```python
from build123d import *

# Parameters (mm, degrees)
PRISM003_DEPTH         = 6
PRISM002_DEPTH         = 6
BOX004_W               = 10
BOX004_H               = 12
BOX004_DEPTH           = 4
BOX003_W               = 35
BOX003_H               = 26.5
BOX003_DEPTH           = 10
BOX002_W               = 70
BOX002_H               = 19
BOX002_DEPTH           = 19
BOX002_PLACEMENT_ANGLE = 30
BOX001_W               = 70
BOX001_H               = 19
BOX001_DEPTH           = 19
BOX001_PLACEMENT_ANGLE = 90.0000000001
BOX_W                  = 70
BOX_H                  = 19
BOX_DEPTH              = 19
BOX_PLACEMENT_ANGLE    = 30
PRISM001_DEPTH         = 25
PRISM_DEPTH            = 25
FILLET_R               = 15
SKETCH001_R            = 2
POCKET_DEPTH           = 782.7773522307
POLARPATTERN_COUNT     = 3
POCKET001_DEPTH        = 3
SKETCH002_R            = 1
POCKET002_DEPTH        = 782.7773522307
POLARPATTERN001_COUNT  = 3
SKETCH004_R            = 1
POCKET003_DEPTH        = 782.7773522307
POLARPATTERN002_COUNT  = 3
POLARPATTERN003_COUNT  = 3
SKETCH005_R            = 1
POCKET004_DEPTH        = 782.7773522307
POLARPATTERN004_COUNT  = 3
POCKET005_DEPTH        = 22.001
SKETCH007_W            = 14
SKETCH007_H            = 9
POCKET006_DEPTH        = 20


with BuildPart() as prism003:
    # Prism003 → Prism003 (new body)
    with BuildSketch(Plane.XY.offset(13)):
        Polygon((106, 0), (-53, 91.7986928012), (-53, -91.7986928012), align=None)
    extrude(amount=PRISM003_DEPTH)


with BuildPart() as cut006:
    # Prism002 → Prism002 (new body)
    with BuildSketch(Plane.XY.offset(13)):
        Polygon((152, 0), (-76, 131.6358613752), (-76, -131.6358613752), align=None)
    extrude(amount=PRISM002_DEPTH)

    # Cut006: cut Prism003
    add(prism003.part, mode=Mode.SUBTRACT)


with BuildPart() as box004:
    # Box004 → Box004 (new body)
    with BuildSketch(Plane(origin=(84, -6, 15), x_dir=(1, 0, 0), z_dir=(0, 0, 1))):
        with Locations((5, 6)):
            Rectangle(BOX004_W, BOX004_H)
    extrude(amount=BOX004_DEPTH)


with BuildPart() as box003:
    # Box003 → Box003 (new body)
    with BuildSketch(Plane(origin=(93, -13.3, 9), x_dir=(1, 0, 0), z_dir=(0, 0, 1))):
        with Locations((17.5, 13.25)):
            Rectangle(BOX003_W, BOX003_H)
    extrude(amount=BOX003_DEPTH)


with BuildPart() as box002:
    # Box002 → Box002 (new body)
    with BuildSketch(Plane.XY):
        with Locations((35, 9.5)):
            Rectangle(BOX002_W, BOX002_H)
    extrude(amount=BOX002_DEPTH)


with BuildPart() as box002_1:
    # Box002 placement: moved
    add(box002.part.moved(Location((7, -82, 0))).rotate(Axis((7, -82, 0), (0, 0, 1)), BOX002_PLACEMENT_ANGLE))


with BuildPart() as box001:
    # Box001 → Box001 (new body)
    with BuildSketch(Plane.XY):
        with Locations((35, 9.5)):
            Rectangle(BOX001_W, BOX001_H)
    extrude(amount=BOX001_DEPTH)


with BuildPart() as box001_1:
    # Box001 placement: moved
    add(box001.part.moved(Location((-55, -35, 0))).rotate(Axis((-55, -35, 0), (0, 0, 1)), BOX001_PLACEMENT_ANGLE))


with BuildPart() as box:
    # Box → Box (new body)
    with BuildSketch(Plane.XY):
        with Locations((35, 9.5)):
            Rectangle(BOX_W, BOX_H)
    extrude(amount=BOX_DEPTH)


with BuildPart() as box_1:
    # Box placement: moved
    add(box.part.moved(Location((-2, 65, 0))).rotate(Axis((-2, 65, 0), (0, 0, -1)), BOX_PLACEMENT_ANGLE))


with BuildPart() as prism001:
    # Prism001 → Prism001 (new body)
    with BuildSketch(Plane.XY.offset(-6)):
        Polygon((95, 0), (-47.5, 82.2724133595), (-47.5, -82.2724133595), align=None)
    extrude(amount=PRISM001_DEPTH)


with BuildPart() as body:
    # Prism → Prism (new body)
    with BuildSketch(Plane.XY.offset(-6)):
        Polygon((165, 0), (-82.5, 142.8941916244), (-82.5, -142.8941916244), align=None)
    extrude(amount=PRISM_DEPTH)

    # Cut: cut Prism001
    add(prism001.part, mode=Mode.SUBTRACT)

    # Cut001: cut Box
    add(box_1.part, mode=Mode.SUBTRACT)

    # Cut002: cut Box001
    add(box001_1.part, mode=Mode.SUBTRACT)

    # Cut003: cut Box002
    add(box002_1.part, mode=Mode.SUBTRACT)

    # Cut004: cut Box003
    add(box003.part, mode=Mode.SUBTRACT)

    # Cut005: cut Box004
    add(box004.part, mode=Mode.SUBTRACT)

    # Cut007: cut Cut006
    add(cut006.part, mode=Mode.SUBTRACT)

    # Fillet
    fillet_edges = [body.edges().sort_by_distance(p)[0] for p in [
        (152, 0, 16),
        (-76, 131.635861, 16),
        (-76, -131.635861, 16),
    ]]
    fillet(fillet_edges, radius=FILLET_R)

    # Sketch001 (on Face1 of BaseFeature) → Pocket (cut, through all)
    with BuildSketch(Plane.XY.offset(19)):
        with Locations((148.549835, 0)):
            Circle(SKETCH001_R)
    pocket = extrude(amount=-POCKET_DEPTH, mode=Mode.SUBTRACT)

    # PolarPattern: Pocket ×3 about axis
    polarpattern_axis = Axis((0, 0, 19), (0, 0, 1))
    for i in range(1, POLARPATTERN_COUNT):
        add(pocket.rotate(polarpattern_axis, i * 360 / POLARPATTERN_COUNT), mode=Mode.SUBTRACT)

    # Sketch003 (on Face14 of PolarPattern) → Pocket001 (cut)
    with BuildSketch(Plane(origin=(0, 0, -6), x_dir=(1, 0, 0), z_dir=(0, 0, -1))):
        Polygon((-70.5, 122.1095819336), (141, 0), (-70.5, -122.1095819336), align=None)
        Polygon((-59.5, -103.0570230503), (-59.5, 103.0570230503), (119, 0), align=None, mode=Mode.SUBTRACT)
    extrude(amount=-POCKET001_DEPTH, mode=Mode.SUBTRACT)

    # Sketch002 (on Face39 of PolarPattern) → Pocket002 (cut, through all)
    with BuildSketch(Plane.XY.offset(19)):
        with Locations((-50.25, 0)):
            Circle(SKETCH002_R)
        with Locations((-50.25, 87.0355530803)):
            Circle(SKETCH002_R)
    pocket002 = extrude(amount=-POCKET002_DEPTH, mode=Mode.SUBTRACT)

    # PolarPattern001: Pocket002 ×3 about axis
    polarpattern001_axis = Axis((0, 0, 19), (0, 0, 1))
    for i in range(1, POLARPATTERN001_COUNT):
        add(pocket002.rotate(polarpattern001_axis, i * 360 / POLARPATTERN001_COUNT), mode=Mode.SUBTRACT)

    # Sketch004 (on Face40 of PolarPattern001) → Pocket003 (cut, through all)
    with BuildSketch(Plane.XY.offset(19)):
        with Locations((84.4115427319, 9)):
            Circle(SKETCH004_R)
        with Locations((84.4115427319, -9)):
            Circle(SKETCH004_R)
    pocket003 = extrude(amount=-POCKET003_DEPTH, mode=Mode.SUBTRACT)

    # PolarPattern002: Pocket003 ×3 about axis
    polarpattern002_axis = Axis((0, 0, 19), (0, 0, 1))
    for i in range(1, POLARPATTERN002_COUNT):
        add(pocket003.rotate(polarpattern002_axis, i * 360 / POLARPATTERN002_COUNT), mode=Mode.SUBTRACT)

    # PolarPattern003: Pocket002 ×3 about axis
    polarpattern003_axis = Axis((0, 0, 19), (0, 0, 1))
    for i in range(1, POLARPATTERN003_COUNT):
        add(pocket002.rotate(polarpattern003_axis, i * 360 / POLARPATTERN003_COUNT), mode=Mode.SUBTRACT)

    # Sketch005 (on Face1 of PolarPattern003) → Pocket004 (cut, through all)
    with BuildSketch(Plane.XY.offset(19)):
        with Locations((-79.25, 0)):
            Circle(SKETCH005_R)
    pocket004 = extrude(amount=-POCKET004_DEPTH, mode=Mode.SUBTRACT)

    # PolarPattern004: Pocket004 ×3 about axis
    polarpattern004_axis = Axis((0, 0, 19), (0, 0, 1))
    for i in range(1, POLARPATTERN004_COUNT):
        add(pocket004.rotate(polarpattern004_axis, i * 360 / POLARPATTERN004_COUNT), mode=Mode.SUBTRACT)

    # Sketch006 (on Face42 of PolarPattern004) → Pocket005 (cut, through all)
    with BuildSketch(Plane(origin=(0, 0, -3), x_dir=(1, 0, 0), z_dir=(0, 0, -1))):
        with BuildLine():
            ThreePointArc((123, 1.5), (121.5, 0), (123, -1.5))
            Line((123, -1.5), (135, -1.5))
            ThreePointArc((135, -1.5), (136.5, 0), (135, 1.5))
            Line((123, 1.5), (135, 1.5))
        make_face()
    extrude(amount=-POCKET005_DEPTH, mode=Mode.SUBTRACT)

    # Sketch007 (on Face3 of Pocket005) → Pocket006 (cut)
    with BuildSketch(Plane(origin=(41.25, -71.4470958122, 0), x_dir=(0.8660254038, 0.5, 0), z_dir=(0.5, -0.8660254038, 0))):
        with Locations((57.9152, 9.460156)):
            Rectangle(SKETCH007_W, SKETCH007_H)
    extrude(amount=-POCKET006_DEPTH, mode=Mode.SUBTRACT)


solid = body.part
```
Work out the finished part from the listing and answer in its coordinate system (mm). A direction names the side the tool comes from. Give positions to 0.01 mm unless a question says otherwise; leave off trailing zeros. Order: outer loops, then holes, each group sorted by start corner. A loop starts at its lowest first (then second) coordinate and runs counter-clockwise, first axis right, second up. Notation, with made-up numbers: (-39.5, 74.25) - (8.5, 74.25) arc R20 ccw to (8.5, 97.25) - close; hole circle Ø2 at (51.25, 52). An arc over 180 degrees is marked (long way). One line per item, written item: value. Start each with the question number.
1. For a pull along Y with two mould halves and no side action, classify faces 1 (the face through (29, 39, -6)), 2 (the face through (-53, 1, 16)), 3 (the face through (39.518, -72.447, 6.325)), 4 (the face through (86, -34, 4.96)) as released by +Y, released by -Y, zero draft, split by the parting line, or undercut.
2. Section A-A, the plane x = 78.5 is taken. Write down the section's boundary in (y, z), then the cut area to 3 significant figures.
3. Consider line 1 (X direction, y = 73, z = 15.25); line 2 (X direction, y = -25, z = 0.5); line 3 (Y direction, x = -50.25, z = 3.75). Determine where each line is inside the solid, lowest interval first.
4. Which of the six approach directions +Z, -Z, +X, -X, +Y, -Y give full straight-line access (tool end or side, diameter ignored) to faces 5 (the face through (80.414, -37.45, 9.397)), 6 (the face through (-65, 0, 0)), 7 (the face through (28, -55, -3))?
5. Section B-B, the plane y = 23 is taken. Write down the section's boundary in (x, z), then the cut area to 4 significant figures.
6. Section D-D, the plane x = -7.5 is taken. Write down the section's boundary in (y, z), then the cut area to 3 significant figures.
7. Each of these flat-tipped pins is pushed along its axis until it touches: pin 1 Ø2 at (x, z) = (106, 11) entering from +Y; pin 2 Ø1.5 at (x, y) = (87.5, 3.5) entering from +Z; pin 3 Ø12 at (x, z) = (1.5, 7) entering from -Y. Where does it stop, or does it pass through?
Filled sheet:
1. face 1: zero draft
1. face 2: undercut
1. face 3: released by -Y
1. face 4: undercut
2. outline: (-49.94, -6) - (-36.08, -6) - (-36.08, -3) - (-23.38, -3) - (-23.38, -6) - (-9.53, -6) - (-9.53, 19) - (-15.88, 19) - (-15.88, 13) - (-26.85, 13) - (-26.85, 4.96) - (-34.14, 4.96) - (-34.14, 13) - (-42.44, 13) - (-42.44, 19) - (-49.94, 19) - close; (9.53, -6) - (23.38, -6) - (23.38, -3) - (36.08, -3) - (36.08, -6) - (49.94, -6) - (49.94, 19) - (42.44, 19) - (42.44, 13) - (15.88, 13) - (15.88, 19) - (9.53, 19) - close
2. area: 1,570 mm²
3. line 1: -82.5 to -76, -53 to -47.5, -31.44 to -20.44, 25.56 to 38.56
3. line 2: -82.5 to -74, -55 to -47.5, 51.7 to 121.7
3. line 3: -124.27 to -88.04, -86.04 to -69.57, -67.63 to -1, 1 to 67.63, 69.57 to 86.04, 88.04 to 124.27
4. face 5: none
4. face 6: +Z
4. face 7: -Z
5. outline: (-82.5, -6) - (-70.5, -6) - (-70.5, -3) - (-59.5, -3) - (-59.5, -6) - (-47.5, -6) - (-47.5, 19) - (-53, 19) - (-53, 13) - (-55, 13) - (-55, 0) - (-74, 0) - (-74, 13) - (-76, 13) - (-76, 19) - (-82.5, 19) - close; (55.16, -6) - (79.16, -6) - (79.16, -3) - (101.16, -3) - (101.16, -6) - (125.16, -6) - (125.16, 19) - (112.16, 19) - (112.16, 13) - (66.16, 13) - (66.16, 19) - (55.16, 19) - close
5. area: 1,865 mm²
6. outline: (-99.59, -6) - (-85.74, -6) - (-85.74, -3) - (-73.03, -3) - (-73.03, -6) - (-59.18, -6) - (-59.18, 19) - (-65.53, 19) - (-65.53, 13) - (-92.09, 13) - (-92.09, 19) - (-99.59, 19) - close; (59.18, -6) - (73.03, -6) - (73.03, -3) - (85.74, -3) - (85.74, -6) - (99.59, -6) - (99.59, 19) - (92.09, 19) - (92.09, 13) - (65.53, 13) - (65.53, 19) - (59.18, 19) - close
6. area: 1,630 mm²
7. pin 1: y = 34.64
7. pin 2: z = 15
7. pin 3: y = -97.86
